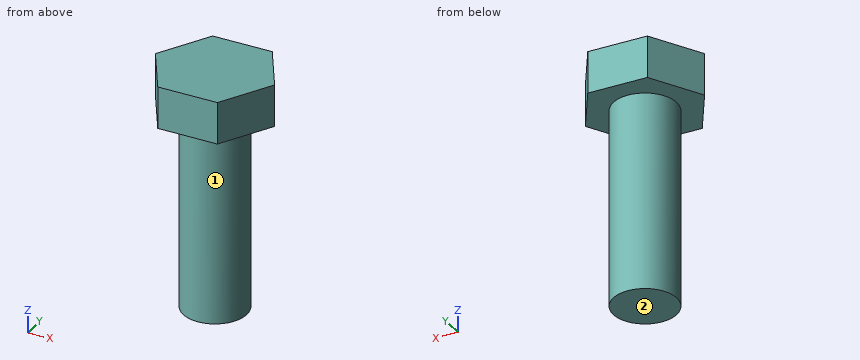
from build123d import *

# Parameters (mm, degrees)
SKETCH1_R      = 4
EXTRUDE1_DEPTH = 25
EXTRUDE2_DEPTH = 5.3


with BuildPart() as part:
    # Sketch1 → Extrude1 (new body)
    with BuildSketch(Plane.XY):
        Circle(SKETCH1_R)
    extrude(amount=-EXTRUDE1_DEPTH)

    # Sketch2 → Extrude2 (add)
    with BuildSketch(Plane.XY):
        Polygon((-3.75277675, 6.5), (-7.505553499, 0), (-3.75277675, -6.5), (3.75277675, -6.5), (7.505553499, 0), (3.75277675, 6.5), align=None)
    extrude(amount=EXTRUDE2_DEPTH)


solid = part.part
Verification items for the finished model (mm, model axes). Face numbers are marked on the shaded views. A direction names the side the tool comes from. Give positions to 0.01 mm unless a question says otherwise; leave off trailing zeros. Write each loop counter-clockwise with the first axis right and the second up, starting at its lowest first coordinate (ties: lowest second). Pieces come first, ordered by that corner, then holes. Notation, with made-up numbers: (23, -17.75) - (68, -17.75) arc R28 ccw to (68, 8.25) - close; hole circle Ø8 at (43.5, -3.75). An arc over 180 degrees is marked (long way). Answer as CSV lines item,"result". Start each with the question number.
1. Sectioned sample at D-D (z = -21). Record the boundary of the cut face in (x, y), then the cut area to 3 significant figures.
2. Sectioned sample at B-B (z = 2.5). Record the boundary of the cut face in (x, y).
3. Thickness scan on line 1 (Z direction, x = -2.25, y = -3.5); line 2 (X direction, y = 0.25, z = -12); line 3 (Y direction, x = 3.5, z = -6.5). Record the ranges inside material, lowest first.
4. Set-up check for the marked faces 1 and 2: record each of +Z, -Z, +X, -X, +Y, -Y from which the full face is reachable in a straight line by a thin tool's end or side.
5. Sectioned sample at A-A (x = 0). Record the boundary of the cut face in (y, z), then the cut area to 3 significant figures.
6. Depth check by flat-ended pin: pin 1 (1.5 mm diameter, centred on y = 4, z = -15, fed in from -X); pin 2 (1 mm diameter, centred on y = 3.5, z = -5.5, fed in from +X). Enter the tip coordinate at first touch or a pass-through.
7. Sectioned sample at C-C (y = -1). Record the boundary of the cut face in (x, z), then the cut area to 3 significant figures.
Derived:
1,outline,"circle Ø8 at (0, 0)"
1,area,"50.3 mm²"
2,outline,"(-7.51, 0) - (-3.75, -6.5) - (3.75, -6.5) - (7.51, 0) - (3.75, 6.5) - (-3.75, 6.5) - close"
3,line 1,"0 to 5.3"
3,line 2,"-3.99 to 3.99"
3,line 3,"-1.94 to 1.94"
4,face 1,"-Z"
4,face 2,"-Z, +X, -X, +Y, -Y"
5,outline,"(-6.5, 0) - (-4, 0) - (-4, -25) - (4, -25) - (4, 0) - (6.5, 0) - (6.5, 5.3) - (-6.5, 5.3) - close"
5,area,"269 mm²"
6,pin 1,"x = -2.33"
6,pin 2,"x = 2.65"
7,outline,"(-6.93, 0) - (-3.87, 0) - (-3.87, -25) - (3.87, -25) - (3.87, 0) - (6.93, 0) - (6.93, 5.3) - (-6.93, 5.3) - close"
7,area,"267 mm²"
